from build123d import *

# Parameters (mm, degrees)
F1_W      = 74
F1_H      = 2.5
F2_DEPTH  = 2.5
F3_DEPTH  = 80
F4_W      = 12
F4_H      = 12
F5_DEPTH  = 3.75
F6_W      = 8.5
F6_H      = 8.5
F7_DEPTH  = 2.5
F9_DEPTH  = 2.5
F10_DEPTH = 7.62
F11_DEPTH = 5.588


with BuildPart() as f2:
    # F1 (on Top) → F2 (new body)
    with BuildSketch(Plane.XY):
        Polygon((37.5, -12.5), (37.5, 12.5), (37, 12.5), (-37, 12.5), (-37.5, 12.5), (-37.5, -12.5), (-12.5, -12.5), align=None)
        with BuildLine():
            Line((37, 12.5), (37.5, 12.5))
            Line((37.5, 12.5), (37.5, -12.5))
            Line((37.5, -12.5), (-12.5, -12.5))
            ThreePointArc((-12.5, -12.5), (-25, -25), (-37.5, -12.5))
            Line((-37.5, -12.5), (-37.5, 12.5))
            Line((-37.5, 12.5), (-37, 12.5))
            Line((-37, 12.5), (-37, 15))
            Line((-37, 15), (-40, 15))
            Line((-40, 15), (-40, -12.5))
            ThreePointArc((-40, -12.5), (-26.2543939042, -27.4474578418), (-10.2098005423, -15))
            Line((-10.2098005423, -15), (40, -15))
            Line((40, -15), (40, 15))
            Line((40, 15), (37, 15))
            Line((37, 15), (37, 12.5))
        make_face()
        with Locations((0, 13.75)):
            Rectangle(F1_W, F1_H)
        with BuildLine():
            ThreePointArc((-37.5, -12.5), (-25, -25), (-12.5, -12.5))
            Line((-12.5, -12.5), (-37.5, -12.5))
        make_face()
    extrude(amount=-F2_DEPTH)

    # F1 (on Top) → F3 (join)
    with BuildSketch(Plane.XY):
        with BuildLine():
            Line((37, 12.5), (37.5, 12.5))
            Line((37.5, 12.5), (37.5, -12.5))
            Line((37.5, -12.5), (-12.5, -12.5))
            ThreePointArc((-12.5, -12.5), (-25, -25), (-37.5, -12.5))
            Line((-37.5, -12.5), (-37.5, 12.5))
            Line((-37.5, 12.5), (-37, 12.5))
            Line((-37, 12.5), (-37, 15))
            Line((-37, 15), (-40, 15))
            Line((-40, 15), (-40, -12.5))
            ThreePointArc((-40, -12.5), (-26.2543939042, -27.4474578418), (-10.2098005423, -15))
            Line((-10.2098005423, -15), (40, -15))
            Line((40, -15), (40, 15))
            Line((40, 15), (37, 15))
            Line((37, 15), (37, 12.5))
        make_face()
        with BuildLine():
            ThreePointArc((-37.5, -12.5), (-25, -25), (-12.5, -12.5))
            Line((-12.5, -12.5), (-37.5, -12.5))
        make_face()
    extrude(amount=F3_DEPTH)

    # F4 (on face) → F5 (cut)
    with BuildSketch(Plane.XY.offset(80)):
        with Locations((-25, -15.5)):
            Rectangle(F4_W, F4_H)
    extrude(amount=-F5_DEPTH, mode=Mode.SUBTRACT)

    # F6 (on face) → F7 (cut, through all)
    with BuildSketch(Plane.XZ.offset(15)):
        with Locations((15, 38.75)):
            Rectangle(F6_W, F6_H)
    extrude(amount=-F7_DEPTH, mode=Mode.SUBTRACT)

    # F8 (on face) → F9 (cut, through all)
    with BuildSketch(Plane.XY):
        with BuildLine():
            Line((16.717254696, -3.1138677411), (13.282745304, -3.1138677411))
            ThreePointArc((13.282745304, -3.1138677411), (15, -3.556), (16.717254696, -3.1138677411))
        make_face()
        with BuildLine():
            ThreePointArc((18.556, 0), (13.191882429, 3.0620004653), (13.282745304, -3.1138677411))
            Line((13.282745304, -3.1138677411), (16.717254696, -3.1138677411))
            ThreePointArc((16.717254696, -3.1138677411), (18.0620004653, -1.808117571), (18.556, 0))
        make_face()
    extrude(amount=-F9_DEPTH, mode=Mode.SUBTRACT)

    # F8 (on face) → F10 (join)
    with BuildSketch(Plane.XY):
        Polygon((15, -6.5991135768), (9.285, -3.2995567884), (9.285, 3.2995567884), (9.285, 9.1138677411), (5, 9.1138677411), (5, -9.1138677411), (25, -9.1138677411), (25, 9.1138677411), (20.715, 9.1138677411), (20.715, 3.2995567884), (20.715, -3.2995567884), align=None)
        Polygon((19, 4.2897125001), (20.715, 3.2995567884), (20.715, 9.1138677411), (19, 9.1138677411), align=None)
        with BuildLine():
            Line((9.285, 3.2995567884), (9.285, -3.2995567884))
            Line((9.285, -3.2995567884), (15, -6.5991135768))
            Line((15, -6.5991135768), (20.715, -3.2995567884))
            Line((20.715, -3.2995567884), (20.715, 3.2995567884))
            Line((20.715, 3.2995567884), (19, 4.2897125001))
            Line((19, 4.2897125001), (19, 3.1138677411))
            Line((19, 3.1138677411), (19, -3.1138677411))
            Line((19, -3.1138677411), (16.717254696, -3.1138677411))
            ThreePointArc((16.717254696, -3.1138677411), (15, -3.556), (13.282745304, -3.1138677411))
            Line((13.282745304, -3.1138677411), (11, -3.1138677411))
            Line((11, -3.1138677411), (11, 3.1138677411))
            Line((11, 3.1138677411), (11, 4.2897125001))
            Line((11, 4.2897125001), (9.285, 3.2995567884))
        make_face()
        Polygon((9.285, 9.1138677411), (9.285, 3.2995567884), (11, 4.2897125001), (11, 9.1138677411), align=None)
    extrude(amount=F10_DEPTH)

    # F8 (on face) → F11 (cut)
    with BuildSketch(Plane.XY):
        with BuildLine():
            Line((9.285, 3.2995567884), (9.285, -3.2995567884))
            Line((9.285, -3.2995567884), (15, -6.5991135768))
            Line((15, -6.5991135768), (20.715, -3.2995567884))
            Line((20.715, -3.2995567884), (20.715, 3.2995567884))
            Line((20.715, 3.2995567884), (19, 4.2897125001))
            Line((19, 4.2897125001), (19, 3.1138677411))
            Line((19, 3.1138677411), (19, -3.1138677411))
            Line((19, -3.1138677411), (16.717254696, -3.1138677411))
            ThreePointArc((16.717254696, -3.1138677411), (15, -3.556), (13.282745304, -3.1138677411))
            Line((13.282745304, -3.1138677411), (11, -3.1138677411))
            Line((11, -3.1138677411), (11, 3.1138677411))
            Line((11, 3.1138677411), (11, 4.2897125001))
            Line((11, 4.2897125001), (9.285, 3.2995567884))
        make_face()
        Polygon((19, 4.2897125001), (20.715, 3.2995567884), (20.715, 9.1138677411), (19, 9.1138677411), align=None)
        Polygon((9.285, 9.1138677411), (9.285, 3.2995567884), (11, 4.2897125001), (11, 9.1138677411), align=None)
    extrude(amount=F11_DEPTH, mode=Mode.SUBTRACT)


solid = f2.part
Geometry check sheet. Reference: the model listing, model coordinates, mm. A direction names the side the tool comes from. Coordinates: 2 decimals unless noted, no trailing zeros. Order: outer loops, then holes, each group sorted by start corner. A loop starts at its lowest first (then second) coordinate and runs counter-clockwise, first axis right, second up. Notation, with made-up numbers: (60, 30) - (65, 30) arc R5 ccw to (65, 38) - close; hole circle Ø5 at (59.5, 25.25). An arc over 180 degrees is marked (long way). Answer in a Markdown table with one row per item. Add a question column.
1) Material ranges on line 1 along X through (y, z) = (-8.5, 65); line 2 along X through (y, z) = (0, -1.65); line 3 along Y through (x, z) = (15, -1.25), recorded low to high. Write a range as [from, to].
2) Gauge pin test, flat ends, axial feed: P1, Ø2, axis at x = -25, y = 6, coming from the +Z side; P2, Ø1.5, axis at y = -23, z = 31.5, coming from the +X side; P3, Ø22, axis at x = 9, y = 7.5, coming from the +Z side; P4, Ø1.5, axis at x = 3, y = -16, coming from the +Z side. Record the tip position at first contact, or that the pin passes through.
3) Set-up check for faces 4 (the flat face through (-25, -17, 76.25)), 5 (the flat face through (-37.5, 0, 39)), 6 (the flat face through (20.715, 3, 3)): record each of +Z, -Z, +X, -X, +Y, -Y from which the full face is reachable in a straight line by a thin tool's end or side.
4) Cross-section at D-D, the plane y = 7. Record the cut outline in (x, z) (3 decimals).
5) Release check for a two-part mould opening along Y. For faces 1 (the flat face through (20, -15, 38)), 2 (the flat face through (-19, -17, 78)), 3 (the flat face through (37.5, 0, 39)) record: +Y half, -Y half, draft (parallel to the pull), parting line (faces both ways), or undercut.
6) Cross-section at A-A, the plane y = -11. Record the cut outline in (x, z), then the cut area to 3 significant figures.
7) Cross-section at C-C, the plane x = 22.5. Record the cut outline in (y, z).
8) Cross-section at B-B, the plane z = 59. Record the cut outline in (x, y).
Check result:
| question | item | result |
|---|---|---|
| 1 | line 1 | x = [-40, -37.5], [37.5, 40] |
| 1 | line 2 | x = [-40, 11.44], [18.56, 40] |
| 1 | line 3 | y = [-15, -3.56], [3.56, 15] |
| 2 | P1 | stops at z = 0 |
| 2 | P2 | stops at x = -13.6 |
| 2 | P3 | stops at z = 7.62 |
| 2 | P4 | passes through |
| 3 | face 4 | +Z, +Y |
| 3 | face 5 | +Z |
| 3 | face 6 | +Y |
| 4 | outline | (-40, -2.5) - (40, -2.5) - (40, 80) - (37.5, 80) - (37.5, 0) - (25, 0) - (25, 7.62) - (19, 7.62) - (19, 5.588) - (20.715, 5.588) - (20.715, 0) - (9.285, 0) - (9.285, 5.588) - (11, 5.588) - (11, 7.62) - (5, 7.62) - (5, 0) - (-37.5, 0) - (-37.5, 80) - (-40, 80) - close |
| 5 | face 1 | -Y half |
| 5 | face 2 | draft |
| 5 | face 3 | undercut |
| 6 | outline | (-40, -2.5) - (40, -2.5) - (40, 80) - (37.5, 80) - (37.5, 0) - (-37.5, 0) - (-37.5, 80) - (-40, 80) - close |
| 6 | area | 600 mm² |
| 7 | outline | (-15, -2.5) - (15, -2.5) - (15, 0) - (9.11, 0) - (9.11, 7.62) - (-9.11, 7.62) - (-9.11, 0) - (-12.5, 0) - (-12.5, 80) - (-15, 80) - close |
| 8 | outline | (-40, -12.5) arc R15 ccw to (-10.21, -15) - (40, -15) - (40, 15) - (37, 15) - (37, 12.5) - (37.5, 12.5) - (37.5, -12.5) - (-37.5, -12.5) - (-37.5, 12.5) - (-37, 12.5) - (-37, 15) - (-40, 15) - close |
